Verification items for the finished model (mm, model axes). Face numbers are marked on the shaded views. A direction names the side the tool comes from. Coordinates: 2 decimals unless noted, no trailing zeros. Loops run counter-clockwise (first coordinate to the right, second up) from the corner with the lowest first, then second, coordinate; pieces in that order, holes last. Notation, with made-up numbers: (7.5, -8.75) - (46.5, -8.75) arc R20 cw to (46.5, 24.25) - close; hole circle Ø9 at (-22.75, 79). An arc over 180 degrees is marked (long way). Answer as CSV lines item,"result". Start each with the question number.
1. Release check for a two-part mould opening along Z. For the marked faces 4, 5, 6 and 7 record: pulls with the +Z half, pulls with the -Z half, needs draft (parallel to the pull), parting line crosses it, or undercut.
2. Cross-section at B-B (z = 0). Enter the section's corners in (x, y).
3. Cross-section at C-C (y = 1.2). Enter the section's corners in (x, z), plus the area to 3 significant figures.
4. Cross-section at D-D (z = -3.5). Enter the section's corners in (x, y).
5. Cross-section at A-A (x = 0). Enter the section's corners in (y, z).
6. Set-up check for the marked faces 1, 2 and 3: record each of +Z, -Z, +X, -X, +Y, -Y from which the full face is reachable in a straight line by a thin tool's end or side.
7. Material ranges on line 1 (Z direction, x = 0, y = 1.35); line 2 (X direction, y = -0.5, z = -1.75); line 3 (Z direction, x = -0.5, y = -1.05), recorded low to high. Write a range as [from, to].
8. Gauge pin test, flat ends, axial feed: P1, Ø0.5, axis at x = -4, z = 2, coming from the +Y side; P2, Ø0.8, axis at y = 2, z = -2, coming from the +X side. Record the tip position at first contact, or that the pin passes through.
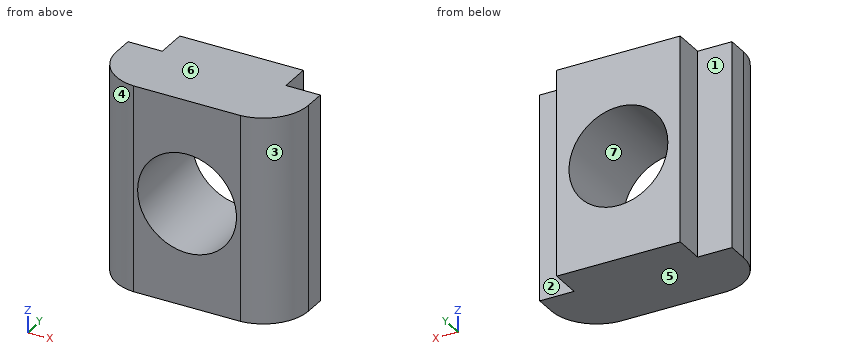
```python
from build123d import *

# Parameters (mm, degrees)
EXTRUDE_1_DEPTH    = 10
HOLE_WIZARD_M6_4_D = 4.8


with BuildPart() as part:
    # 草图1 → 凸台-拉伸1 (new body)
    with BuildSketch(Plane.XY):
        with BuildLine():
            Line((3, 3), (-3, 3))
            Line((-3, 3), (-3, 1.5))
            Line((-3, 1.5), (-4.666746731, 1.5))
            Line((-4.666746731, 1.5), (-4.666746731, 0.5))
            ThreePointArc((-4.666746731, 0.5), (-4.068683171, -1.006990331), (-2.6, -1.69377241))
            Line((-2.6, -1.69377241), (2.6, -1.69377241))
            ThreePointArc((2.6, -1.69377241), (4.068683171, -1.006990331), (4.666746731, 0.5))
            Line((4.666746731, 0.5), (4.666746731, 1.5))
            Line((4.666746731, 1.5), (3, 1.5))
            Line((3, 1.5), (3, 3))
        make_face()
    extrude(amount=EXTRUDE_1_DEPTH)

    # M6 螺纹孔4 (through all)
    with Locations(Plane(origin=(0, 3, 0), x_dir=(1, 0, 0), z_dir=(0, 1, 0))):
        with Locations((0, -5)):
            Hole(HOLE_WIZARD_M6_4_D / 2)


with BuildPart() as part_1:
    # Move Body 1: moved
    add(part.part.moved(Location((0, 0, -5))))


solid = part_1.part
```
Values follow:
1,face 4,"needs draft"
1,face 5,"pulls with the -Z half"
1,face 6,"pulls with the +Z half"
1,face 7,"undercut"
2,outline,"(-4.67, 0.5) arc R2.2 ccw to (-2.6, -1.69) - (-2.4, -1.69) - (-2.4, 3) - (-3, 3) - (-3, 1.5) - (-4.67, 1.5) - close; (2.4, -1.69) - (2.6, -1.69) arc R2.2 ccw to (4.67, 0.5) - (4.67, 1.5) - (3, 1.5) - (3, 3) - (2.4, 3) - close"
3,outline,"(-4.67, -5) - (4.67, -5) - (4.67, 5) - (-4.67, 5) - close; hole circle Ø4.8 at (0, 0)"
3,area,"75.2 mm²"
4,outline,"(-4.67, 0.5) arc R2.2 ccw to (-2.6, -1.69) - (2.6, -1.69) arc R2.2 ccw to (4.67, 0.5) - (4.67, 1.5) - (3, 1.5) - (3, 3) - (-3, 3) - (-3, 1.5) - (-4.67, 1.5) - close"
5,outline,"(-1.69, -5) - (3, -5) - (3, -2.4) - (-1.69, -2.4) - close; (-1.69, 2.4) - (3, 2.4) - (3, 5) - (-1.69, 5) - close"
6,face 1,"+Z, -Z, -X, +Y"
6,face 2,"+Z, -Z, +X, +Y"
6,face 3,"+Z, -Z, +X, -Y"
7,line 1,"z = [-5, -2.4], [2.4, 5]"
7,line 2,"x = [-4.43, -1.64], [1.64, 4.43]"
7,line 3,"z = [-5, -2.35], [2.35, 5]"
8,P1,"stops at y = 1.5"
8,P2,"stops at x = 3"
